from build123d import *

# Parameters (mm, degrees)
BOSS_EXTRUDE1_DEPTH = 2.8
FILLET1_R           = 9
FILLET2_R           = 5


with BuildPart() as part:
    # Sketch1 → Boss-Extrude1 (new body)
    with BuildSketch(Plane.XY):
        with BuildLine():
            Line((3.163348562, 36.5), (76.75, 36.5))
            Line((76.75, 36.5), (76.75, -36.5))
            Line((76.75, -36.5), (-76.75, -36.5))
            Line((-76.75, -36.5), (-76.75, 36.5))
            Line((-76.75, 36.5), (-8.836651438, 36.5))
            ThreePointArc((-8.836651438, 36.5), (-2.836651438, 42.5), (3.163348562, 36.5))
        make_face()
    extrude(amount=BOSS_EXTRUDE1_DEPTH)

    # Fillet1
    fillet1_edges = [part.edges().sort_by_distance(p)[0] for p in [
        (76.75, -36.5, 1.4),
        (-76.75, -36.5, 1.4),
    ]]
    fillet(fillet1_edges, radius=FILLET1_R)

    # Fillet2
    fillet2_edges = [part.edges().sort_by_distance(p)[0] for p in [
        (-76.75, 36.5, 1.4),
        (76.75, 36.5, 1.4),
    ]]
    fillet(fillet2_edges, radius=FILLET2_R)


solid = part.part
Here's how the part is built. I have some questions about the finished solid (model axes, mm). A direction names the side the tool comes from. Coordinates: 2 decimals unless noted, no trailing zeros. Write each loop counter-clockwise with the first axis right and the second up, starting at its lowest first coordinate (ties: lowest second). Pieces come first, ordered by that corner, then holes. Notation, with made-up numbers: (-23, 85) - (14, 85) arc R24 cw to (14, 99) - close; hole circle Ø9 at (49.5, 76.5). An arc over 180 degrees is marked (long way). Use one line per item in the form item = value.
1) I'm going to push a flat-ended pin straight in: P1, Ø0.8, axis at x = 33, z = 1.5, coming from the +Y side. Where does the tip first touch, or does it pass through?
Solved:
P1 = 36.5
2) I need wall thicknesses on line 1 (Y direction, x = 10, z = 0.4); line 2 (Y direction, x = -3, z = 2); line 3 (X direction, y = 35, z = 2.6). Which ranges of each line are inside material? Lowest first, please.
Solved:
line_1 = -36.5 to 36.5
line_2 = -36.5 to 42.5
line_3 = -75.32 to 75.32
3) On a 3-axis mill with a long thin cutter (end or side, diameter ignored), from which of +Z, -Z, +X, -X, +Y, -Y can I reach the whole of each face in a straight line? I mean faces 1 (the flat face through (-76.75, 2, 1)), 2 (the flat face through (37, 36.5, 1)), 3 (the flat face through (-41, 36.5, 1)). Say none if no direction works.
Solved:
face_1 = +Z, -Z, -X, +Y, -Y
face_2 = +Z, -Z, +X, +Y
face_3 = +Z, -Z, -X, +Y
4) Suppose I cut it at A-A, the plane z = 2. Write out the boundary of the cut face in (x, y).
Solved:
outline = (-76.75, -27.5) arc R9 ccw to (-67.75, -36.5) - (67.75, -36.5) arc R9 ccw to (76.75, -27.5) - (76.75, 31.5) arc R5 ccw to (71.75, 36.5) - (3.16, 36.5) arc R6 ccw to (-8.84, 36.5) - (-71.75, 36.5) arc R5 ccw to (-76.75, 31.5) - close
5) Suppose I cut it at B-B, the plane x = 25. Write out the boundary of the cut face in (y, z).
Solved:
outline = (-36.5, 0) - (36.5, 0) - (36.5, 2.8) - (-36.5, 2.8) - close
